Part model, mm, in its own coordinate system. A direction names the side the tool comes from. Give positions to 0.01 mm unless a question says otherwise; leave off trailing zeros. Use a Markdown table: item, result. Add a question column.
from build123d import *

# Parameters (mm, degrees)
F3_W           = 74.675485
F3_H           = 46.419974
F0_DEPTH       = 100.705625
F1_R           = 5
F2_D           = 5
F2_CBORE_D     = 10
F2_CBORE_DEPTH = 5


with BuildPart() as f0:
    # F3 (on Front) → F0 (new body)
    with BuildSketch(Plane.XZ):
        with Locations((37.337742, 23.209987)):
            Rectangle(F3_W, F3_H)
    extrude(amount=F0_DEPTH)

    # F1
    f1_edges = [f0.edges().sort_by_distance(p)[0] for p in [
        (74.675485, -50.352813, 46.419974),
        (37.337743, -100.705625, 46.419974),
        (37.337743, 0, 46.419974),
        (0, -50.352813, 46.419974),
    ]]
    fillet(f1_edges, radius=F1_R)

    # F2 (through all)
    with Locations(Plane(origin=(0, 0, 0), x_dir=(1, 0, 0), z_dir=(0, 0, -1))):
        with Locations((37.771776, 66.144571)):
            CounterBoreHole(F2_D / 2, F2_CBORE_D / 2, F2_CBORE_DEPTH)


solid = f0.part
1. Tool access for faces 5 (the cylindrical face through (36.688, -61.263, 2.465)), 6 (the flat face through (74.675, -50, 20)): list every direction of +Z, -Z, +X, -X, +Y, -Y with a clear straight run to the whole face (end or side of a thin tool).
2. Drill centre lines: probe 1 along Z at (x, y) = (71, -34); probe 2 along X at (y, z) = (-12, 44); probe 3 along Z at (x, y) = (16.5, -4). Where is each one in solid material? Low to high. Write a range as [from, to].
3. Flat gauge pins, fed straight in: pin 1 (3 mm diameter, centred on x = 37.77, y = -66.14, fed in from +Z); pin 2 (6 mm diameter, centred on x = 37.77, y = -66.14, fed in from -Z). Where does each tip first touch, or does it go through?
4. Mould opens along Y. For faces 1 (the flat face through (35, -65, 5)), 2 (the cylindrical face through (37.86, -1.5, 44.99)), 3 (the flat face through (37, -50, 0)), 4 (the flat face through (37, -100.706, 21)) say: released by +Y, released by -Y, zero draft, split by the parting line, or undercut.
A:
| question | item | result |
|---|---|---|
| 1 | face 5 | -Z |
| 1 | face 6 | +Z, -Z, +X, +Y, -Y |
| 2 | probe 1 | z = [0, 46.24] |
| 2 | probe 2 | x = [0.72, 73.96] |
| 2 | probe 3 | z = [0, 46.32] |
| 3 | pin 1 | passes through |
| 3 | pin 2 | stops at z = 5 |
| 4 | face 1 | undercut |
| 4 | face 2 | released by +Y |
| 4 | face 3 | zero draft |
| 4 | face 4 | released by -Y |
